Here's the drawing with two shaded views (mm, measured from the low corner). I have some questions. Give positions to 0.01 mm unless a question says otherwise; leave off trailing zeros. Order: outer loops, then holes, each group sorted by start corner. A loop starts at its lowest first (then second) coordinate and runs counter-clockwise, first axis right, second up. Notation, with made-up numbers: (44, 74.5) - (58, 74.5) arc R12 ccw to (58, 82.5) - close; hole circle Ø1 at (7.5, -39.5). An arc over 180 degrees is marked (long way). Use one line per item in the form item = value. Start each with the question number.
1) Suppose I cut it at A-A, the plane x = 10. Write out the boundary of the cut face in (y, z).
2) Suppose I cut it at D-D, the plane z = 50. Write out the boundary of the cut face in (x, y) (3 decimals).
3) Suppose I cut it at C-C, the plane z = 90. Write out the boundary of the cut face in (x, y).
4) Please list where these lines run through material, in increasing order: probe 1 along Z at (x, y) = (10, 5.25); probe 2 along X at (y, z) = (5, 9).
5) Suppose I cut it at B-B, the plane y = 3. Write out the boundary of the cut face in (x, z) (3 decimals), and give its area (3 significant figures).
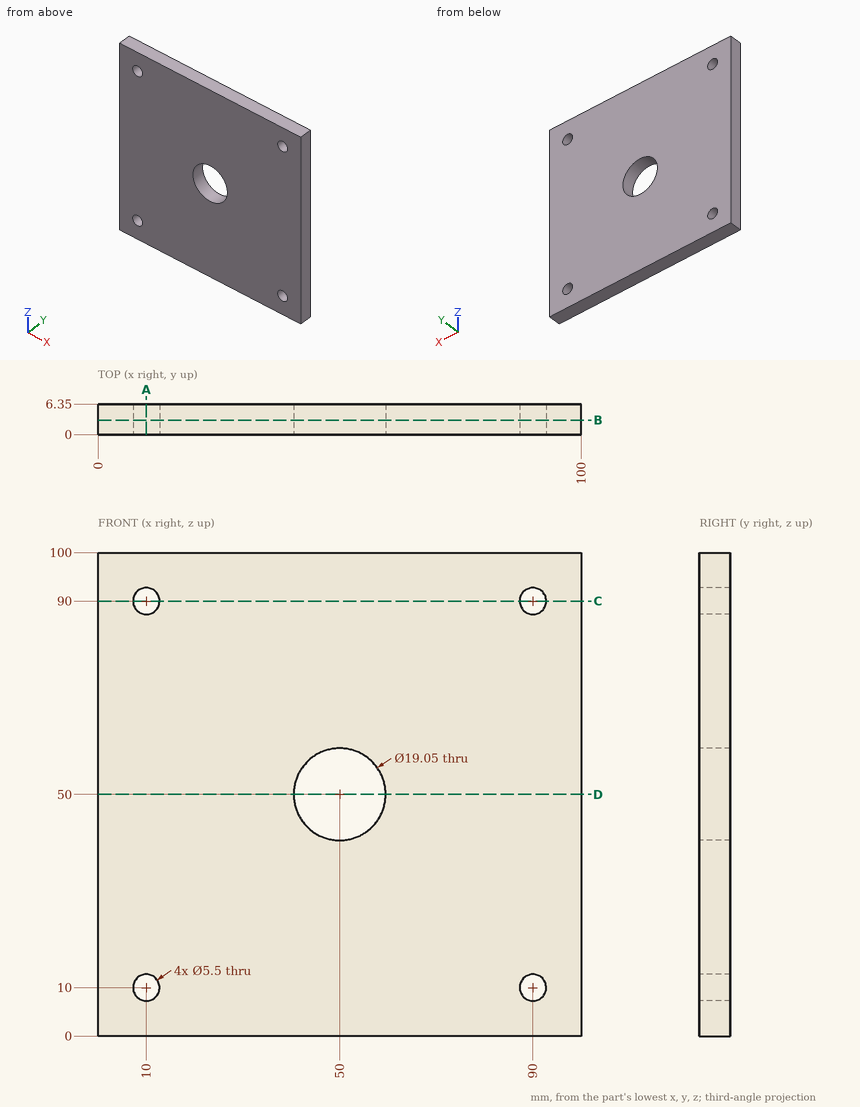
Result sheet:
q1.outline = (0, 0) - (6.35, 0) - (6.35, 7.25) - (0, 7.25) - close; (0, 12.75) - (6.35, 12.75) - (6.35, 87.25) - (0, 87.25) - close; (0, 92.75) - (6.35, 92.75) - (6.35, 100) - (0, 100) - close
q2.outline = (0, 0) - (40.475, 0) - (40.475, 6.35) - (0, 6.35) - close; (59.525, 0) - (100, 0) - (100, 6.35) - (59.525, 6.35) - close
q3.outline = (0, 0) - (7.25, 0) - (7.25, 6.35) - (0, 6.35) - close; (12.75, 0) - (87.25, 0) - (87.25, 6.35) - (12.75, 6.35) - close; (92.75, 0) - (100, 0) - (100, 6.35) - (92.75, 6.35) - close
q4.probe_1 = 0 to 7.25, 12.75 to 87.25, 92.75 to 100
q4.probe_2 = 0 to 7.44, 12.56 to 87.44, 92.56 to 100
q5.outline = (0, 0) - (100, 0) - (100, 100) - (0, 100) - close; hole circle Ø5.5 at (10, 10); hole circle Ø5.5 at (10, 90); hole circle Ø19.05 at (50, 50); hole circle Ø5.5 at (90, 10); hole circle Ø5.5 at (90, 90)
q5.area = 9,620 mm²
